Here's the drawing with two shaded views (mm, measured from the low corner). I have some questions. Coordinates: 2 decimals unless noted, no trailing zeros. Write each loop counter-clockwise with the first axis right and the second up, starting at its lowest first coordinate (ties: lowest second). Pieces come first, ordered by that corner, then holes. Notation, with made-up numbers: M -18,17 L 34,17 A22 cw 34,45 Z; hole C 69,77.5 d10. An arc over 180 degrees is marked long. Answer as CSV lines item,"result". Start each with the question number.
Item 1: We'd pull the mould along X, two halves only. Please class the marked faces 1 and 2: +X half, -X half, draft (parallel to the pull), parting line (faces both ways), or undercut.
Item 2: If I drill on line 1 along Y through (x, z) = (21, 120.5); line 2 along X through (y, z) = (22, 45); line 3 along Y through (x, z) = (5.5, 187), over which ranges is the centre line in solid material (lowest first)? Write a range as [from, to].
Item 3: I'm going to push flat-ended pins straight in: P1, Ø3, axis at y = 13, z = 93, coming from the -X side; P2, Ø1.5, axis at x = 24.5, z = 156, coming from the -Y side; P3, Ø6, axis at y = 23, z = 101, coming from the -X side. Where does each tip first touch, or does it pass through?
Item 4: Suppose I cut it at B-B, the plane x = 10. Write out the boundary of the cut face in (y, z), and give its area (3 significant figures).
Item 5: Suppose I cut it at C-C, the plane z = 113. Write out the boundary of the cut face in (x, y), and give its area (3 significant figures).
Item 6: Suppose I cut it at A-A, the plane y = 21. Write out the boundary of the cut face in (x, z), and give its area (3 significant figures).
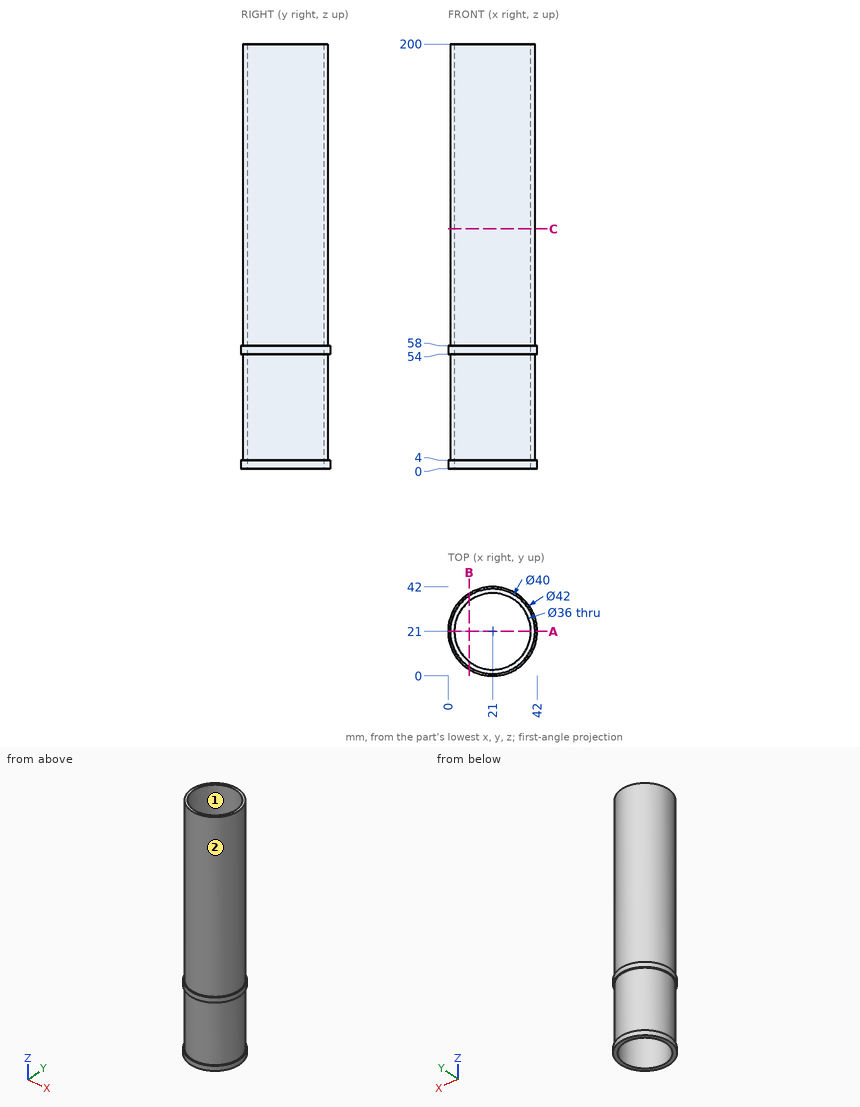
Ans:
1,face 1,"undercut"
1,face 2,"parting line"
2,line 1,"y = [1, 3], [39, 41]"
2,line 2,"x = [1.03, 3.03], [38.97, 40.97]"
2,line 3,"y = [8.36, 11.85], [30.15, 33.64]"
3,P1,"stops at x = 2.09"
3,P2,"stops at y = 1.19"
3,P3,"stops at x = 1"
4,outline,"M 3.11,0 L 6.75,0 L 6.75,200 L 4.3,200 L 4.3,58 L 3.11,58 L 3.11,54 L 4.3,54 L 4.3,4 L 3.11,4 Z; M 35.25,0 L 38.89,0 L 38.89,4 L 37.7,4 L 37.7,54 L 38.89,54 L 38.89,58 L 37.7,58 L 37.7,200 L 35.25,200 Z"
4,area,"1,000 mm^2"
5,outline,"C 21,21 d40; hole C 21,21 d36"
5,area,"239 mm^2"
6,outline,"M 0,0 L 3,0 L 3,200 L 1,200 L 1,58 L 0,58 L 0,54 L 1,54 L 1,4 L 0,4 Z; M 39,0 L 42,0 L 42,4 L 41,4 L 41,54 L 42,54 L 42,58 L 41,58 L 41,200 L 39,200 Z"
6,area,"816 mm^2"
